```python
from build123d import *

# Parameters (mm, degrees)
PAD005_DEPTH    = 4
POCKET010_DEPTH = 49.172573
POCKET011_DEPTH = 49.172573


with BuildPart() as part:
    # Sketch016 → Pad005 (new body)
    with BuildSketch(Plane.XZ):
        Polygon((-21.371573, 17.5), (-30, 17.5), (-30, -7.5), (-21.371573, -16.128427), (-21.371573, -13.3), (21.08873, -13.3), (27.8, -6.58873), (27.8, 15.3), (-21.371573, 15.3), align=None)
    extrude(amount=PAD005_DEPTH)

    # Sketch017 (on DatumPlane) → Pocket010 (cut, through all)
    with BuildSketch(Plane(origin=(-21.371573, 0, 0), x_dir=(0, 0, -1), z_dir=(-1, 0, 0))):
        Polygon((13.3, 0), (11.3, 2), (11.3, 4), (13.3, 4), align=None)
    extrude(amount=-POCKET010_DEPTH, mode=Mode.SUBTRACT)

    # Sketch018 (on DatumPlane) → Pocket011 (cut, through all)
    with BuildSketch(Plane(origin=(-21.371573, 0, 0), x_dir=(0, 0, -1), z_dir=(-1, 0, 0))):
        Polygon((-15.3, 4), (-15.3, 0), (-13.3, 2), (-13.3, 4), align=None)
    extrude(amount=-POCKET011_DEPTH, mode=Mode.SUBTRACT)

    # Sketch020 (on DatumPlane) → Groove (revolve, cut)
    with BuildSketch(Plane(origin=(-26, -41, 1), x_dir=(1, 0, 0), z_dir=(0, 0, -1))):
        Polygon((0, -41), (0, -37), (3, -37), (3, -40), (1.7, -40), (1.7, -41), align=None)
    revolve(axis=Axis((-26, -41, 1), (0, -1, 0)), mode=Mode.SUBTRACT)


solid = part.part
```
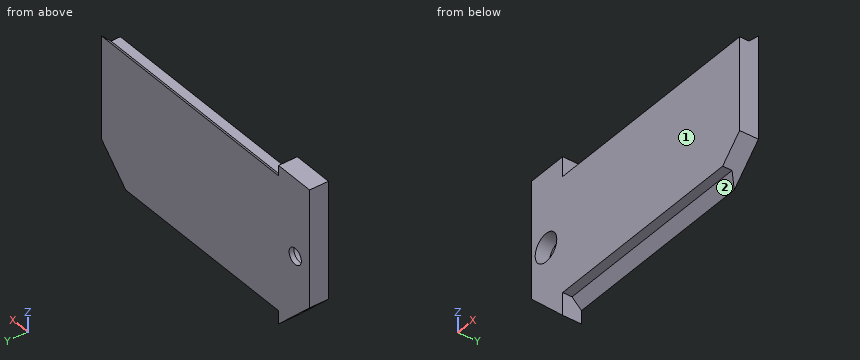
Read the model definition and answer for the solid it produces. Units are mm, in the model's axes. Face numbers are marked on the shaded views. A direction names the side the tool comes from. Round coordinates to 2 decimals unless told otherwise and drop trailing zeros. Write each loop counter-clockwise with the first axis right and the second up, starting at its lowest first coordinate (ties: lowest second). Pieces come first, ordered by that corner, then holes. Notation, with made-up numbers: (-39.75, -9.75) -> (-6.75, -9.75) arc R18 cw to (-6.75, -2.75) -> close; hole circle Ø4 at (-7.5, 18). An arc over 180 degrees is marked (long way). Answer in a Markdown table with one row per item. Add a question column.
1) Given P1, Ø2, axis at y = -1.5, z = -14, coming from the +X side; P2, Ø3.5, axis at x = -26, z = 1, coming from the -Y side; P3, Ø2, axis at x = 11, y = -2.5, coming from the -Z side, each flat-ended and moving along its own axis, determine where each tip first touches the part or whether it passes through.
2) Which of the six approach directions +Z, -Z, +X, -X, +Y, -Y give full straight-line access (tool end or side, diameter ignored) to the marked faces 1 and 2?
3) Find section A-A, the plane z = 1. Determine the outline of the cut face in (x, y), and give its area (3 significant figures).
4) Find section C-C, the plane y = -2.6. Determine the outline of the cut face in (x, z).
5) Consider line 1 (X direction, y = -2.15, z = 15); line 2 (Z direction, x = -26, y = -2.4); line 3 (Z direction, x = -26, y = -0.4). Determine where each line is inside the solid, lowest interval first.
6) Find section B-B, the plane x = -26. Determine the outline of the cut face in (y, z).
7) Find section D-D, the plane z = 14. Determine the outline of the cut face in (x, y), and give its area (3 significant figures).
Findings below:
| question | item | result |
|---|---|---|
| 1 | P1 | x = -21.37 |
| 1 | P2 | y = -1 |
| 1 | P3 | z = -11.8 |
| 2 | face 1 | +Z, -Z, +X, -X, -Y |
| 2 | face 2 | -Z, +X, -Y |
| 3 | outline | (-30, -4) -> (-29, -4) -> (-29, -1) -> (-27.7, -1) -> (-27.7, 0) -> (-30, 0) -> close; (-24.3, -1) -> (-23, -1) -> (-23, -4) -> (27.8, -4) -> (27.8, 0) -> (-24.3, 0) -> close |
| 3 | area | 210 mm² |
| 4 | outline | (-30, -7.5) -> (-21.37, -16.13) -> (-21.37, -11.3) -> (23.09, -11.3) -> (27.8, -6.59) -> (27.8, 13.3) -> (-21.37, 13.3) -> (-21.37, 17.5) -> (-30, 17.5) -> close; hole circle Ø6 at (-26, 1) |
| 5 | line 1 | -30 to -21.37 |
| 5 | line 2 | -11.5 to -2, 4 to 17.5 |
| 5 | line 3 | -11.5 to -0.7, 2.7 to 17.5 |
| 6 | outline | (-4, -11.5) -> (0, -11.5) -> (0, -0.7) -> (-1, -0.7) -> (-1, -2) -> (-4, -2) -> close; (-4, 4) -> (-1, 4) -> (-1, 2.7) -> (0, 2.7) -> (0, 17.5) -> (-4, 17.5) -> close |
| 7 | outline | (-30, -4) -> (-21.37, -4) -> (-21.37, -1.3) -> (27.8, -1.3) -> (27.8, 0) -> (-30, 0) -> close |
| 7 | area | 98.4 mm² |
